For this review, use the dimensioned drawing (mm, ordinates from the lowest corner) and the shaded views. Round coordinates to 2 decimals unless told otherwise and drop trailing zeros. Loops run counter-clockwise (first coordinate to the right, second up) from the corner with the lowest first, then second, coordinate; pieces in that order, holes last. Notation, with made-up numbers: (5, 10) -> (30, 10) arc R13 ccw to (30, 35) -> close; hole circle Ø2 at (68.25, -2). An arc over 180 degrees is marked (long way). Use one line per item in the form item = value. Start each with the question number.
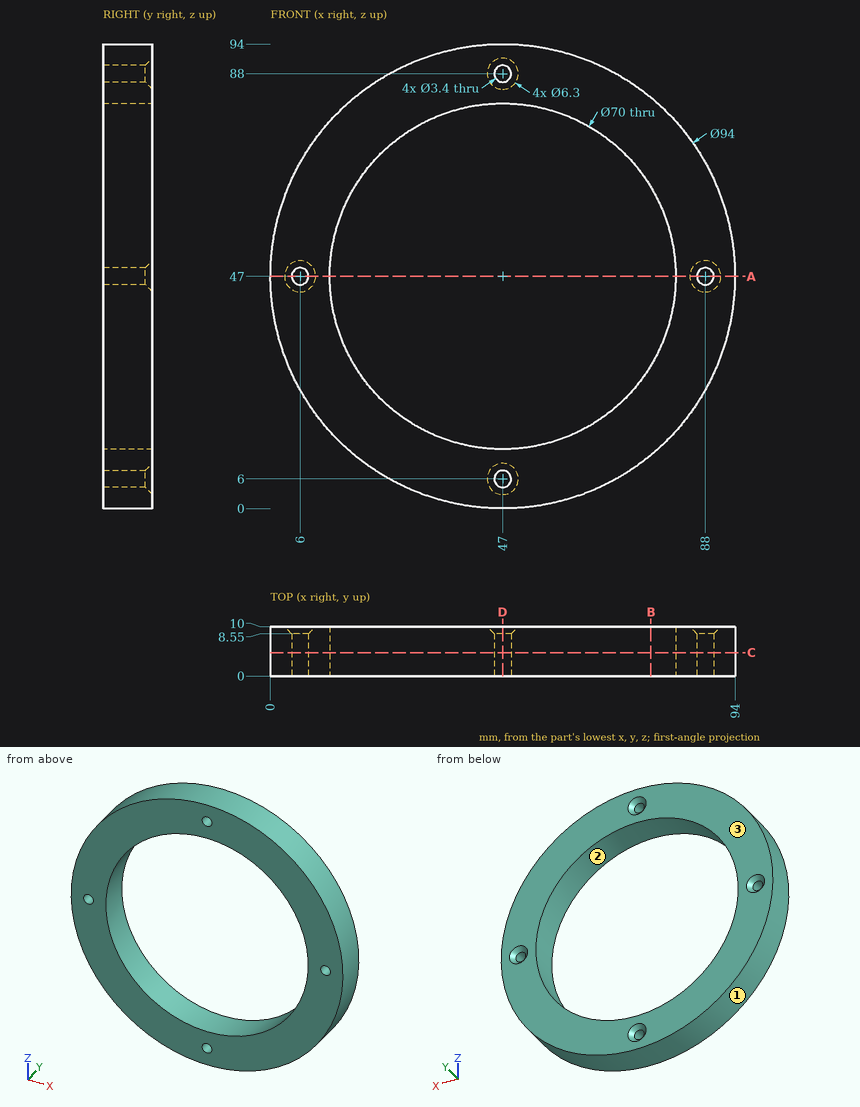
Item 1: Draft analysis for pull direction X (two halves, no side actions). For the marked faces 1, 2 and 3, state which applies: +X half, -X half, draft (parallel to the pull), parting line (faces both ways), or undercut.
Item 2: Take a section at C-C on y = 4.75. Give the boundary of the cut face in (x, z).
Item 3: Wall thickness on line 1 (X direction, y = 2.5, z = 47); line 2 (Z direction, x = 6.5, y = 6.25); line 3 (X direction, y = 6.5, z = 15): over which ranges is each line inside the solid? List them lowest first.
Item 4: For P1, Ø3, axis at x = 51, y = 2.5, coming from the -Z side; P2, Ø4, axis at x = 47, z = 88, coming from the +Y side; P3, Ø3, axis at y = 4.5, z = 50, coming from the -X side; P4, Ø3, axis at x = 47, z = 6, coming from the +Y side (1 decimal), all flat-tipped, find the tip position at first contact; note any pin that passes through.
Item 5: Take a section at B-B on x = 77. Give the boundary of the cut face in (y, z).
Item 6: Take a section at D-D on x = 47. Give the boundary of the cut face in (y, z).
Item 7: Take a section at A-A on z = 47. Give the boundary of the cut face in (x, y), plus the area to 3 significant figures.
Results:
q1.face_1 = parting line
q1.face_2 = undercut
q1.face_3 = draft
q2.outline = circle Ø94 at (47, 47); hole circle Ø3.4 at (6, 47); hole circle Ø70 at (47, 47); hole circle Ø3.4 at (47, 6); hole circle Ø3.4 at (47, 88); hole circle Ø3.4 at (88, 47)
q3.line_1 = 0 to 4.3, 7.7 to 12, 82 to 86.3, 89.7 to 94
q3.line_2 = 23.15 to 45.38, 48.62 to 70.85
q3.line_3 = 12.58 to 32.82, 61.18 to 81.42
q4.P1 = 0.07
q4.P2 = 8.85
q4.P3 = 0.02
q4.P4 = through
q5.outline = (0, 10.82) -> (10, 10.82) -> (10, 28.97) -> (0, 28.97) -> close; (0, 65.03) -> (10, 65.03) -> (10, 83.18) -> (0, 83.18) -> close
q6.outline = (0, 0) -> (10, 0) -> (10, 2.85) -> (8.55, 4.3) -> (0, 4.3) -> close; (0, 7.7) -> (8.55, 7.7) -> (10, 9.15) -> (10, 12) -> (0, 12) -> close; (0, 82) -> (10, 82) -> (10, 84.85) -> (8.55, 86.3) -> (0, 86.3) -> close; (0, 89.7) -> (8.55, 89.7) -> (10, 91.15) -> (10, 94) -> (0, 94) -> close
q7.outline = (0, 0) -> (4.3, 0) -> (4.3, 8.55) -> (2.85, 10) -> (0, 10) -> close; (7.7, 0) -> (12, 0) -> (12, 10) -> (9.15, 10) -> (7.7, 8.55) -> close; (82, 0) -> (86.3, 0) -> (86.3, 8.55) -> (84.85, 10) -> (82, 10) -> close; (89.7, 0) -> (94, 0) -> (94, 10) -> (91.15, 10) -> (89.7, 8.55) -> close
q7.area = 168 mm2
